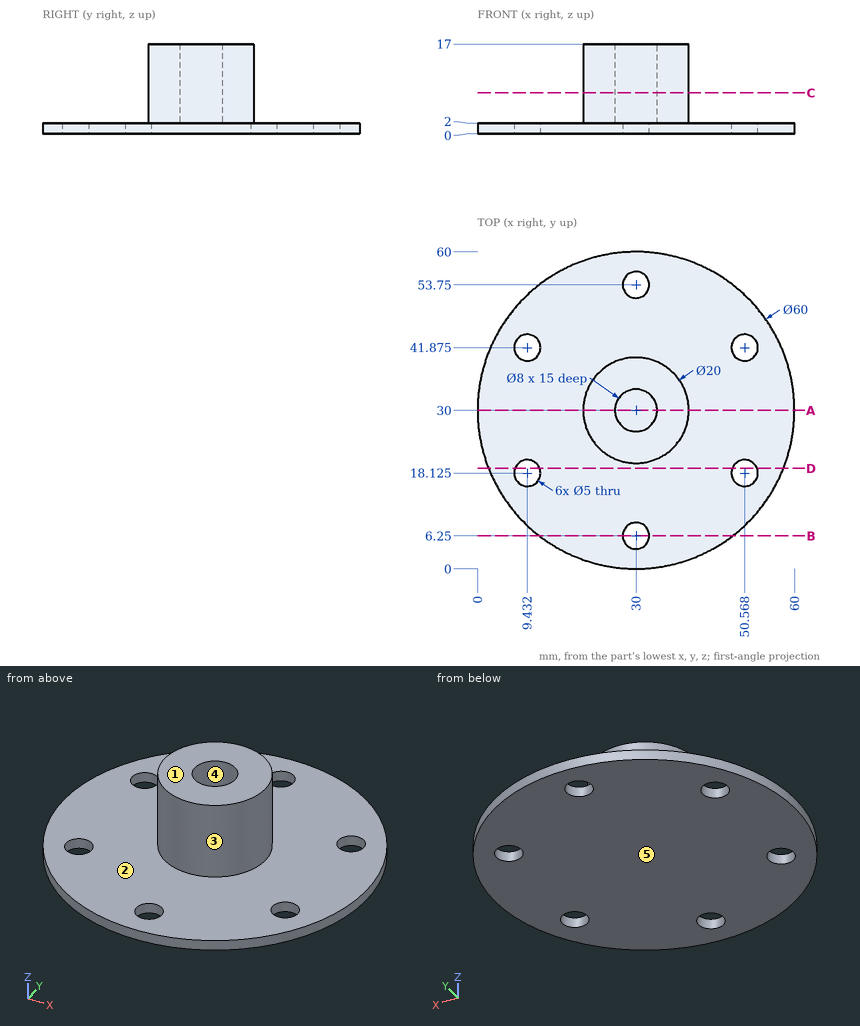
Here's the drawing with two shaded views (mm, measured from the low corner). I have some questions. A direction names the side the tool comes from. Round coordinates to 2 decimals unless told otherwise and drop trailing zeros. Write each loop counter-clockwise with the first axis right and the second up, starting at its lowest first coordinate (ties: lowest second). Pieces come first, ordered by that corner, then holes. Notation, with made-up numbers: M -32,-14.5 L -20,-14.5 A29 ccw -20,9.5 Z; hole C -18,65.5 d8. An arc over 180 degrees is marked long. Write each question's results on one line, items separated by ' | '. Start each with the question number.
1. Imagine slicing it at C-C on z = 7.75. List the corners of the cut face in (x, y) for me.
2. Thinking about a two-plate mould opening in Y: for the marked faces 3, 4 and 5, which applies, +Y half, -Y half, draft (parallel to the pull), parting line (faces both ways), or undercut?
3. I need wall thicknesses on L1, parallel to Z at x = 20.5, y = 15; L2, parallel to Y at x = 30, z = 9.75; L3, parallel to X at y = 29.5, z = 5.25. Which ranges of each line are inside material? Lowest first, please. Write a range as from..to.
4. On a 3-axis mill with a long thin cutter (end or side, diameter ignored), from which of +Z, -Z, +X, -X, +Y, -Y can I reach the whole of each face in a straight line? I mean the marked faces 1 and 2. Say none if no direction works.
5. Imagine slicing it at D-D on y = 19. List the corners of the cut face in (x, z) for me, and give its area (3 significant figures).
6. Imagine slicing it at B-B on y = 6.25. List the corners of the cut face in (x, z) for me, and give its area (3 significant figures).
7. Imagine slicing it at A-A on y = 30. List the corners of the cut face in (x, z) for me, and give its area (3 significant figures).
8. I'm going to push flat-ended pins straight in: pin 1 Ø10 at (x, z) = (33, 2.5) entering from -Y; pin 2 Ø4 at (x, z) = (31, 7) entering from -Y; pin 3 Ø10 at (y, z) = (27.5, 11) entering from -X. Where does each tip first touch, or does it pass through?
Result sheet:
1) outline: C 30,30 d20; hole C 30,30 d8
2) face 3: parting line | face 4: undercut | face 5: draft
3) L1: z = 0..2 | L2: y = 20..26, 34..40 | L3: x = 20.01..26.03, 33.97..39.99
4) face 1: +Z, +X, -X, +Y, -Y | face 2: +Z
5) outline: M 2.09,0 L 7.09,0 L 7.09,2 L 2.09,2 Z; M 11.77,0 L 48.23,0 L 48.23,2 L 11.77,2 Z; M 52.91,0 L 57.91,0 L 57.91,2 L 52.91,2 Z | area: 92.9 mm^2
6) outline: M 11.67,0 L 27.5,0 L 27.5,2 L 11.67,2 Z; M 32.5,0 L 48.33,0 L 48.33,2 L 32.5,2 Z | area: 63.3 mm^2
7) outline: M 0,0 L 60,0 L 60,2 L 40,2 L 40,17 L 34,17 L 34,2 L 26,2 L 26,17 L 20,17 L 20,2 L 0,2 Z | area: 300 mm^2
8) pin 1: stops at y = 0 | pin 2: stops at y = 20 | pin 3: stops at x = 20
